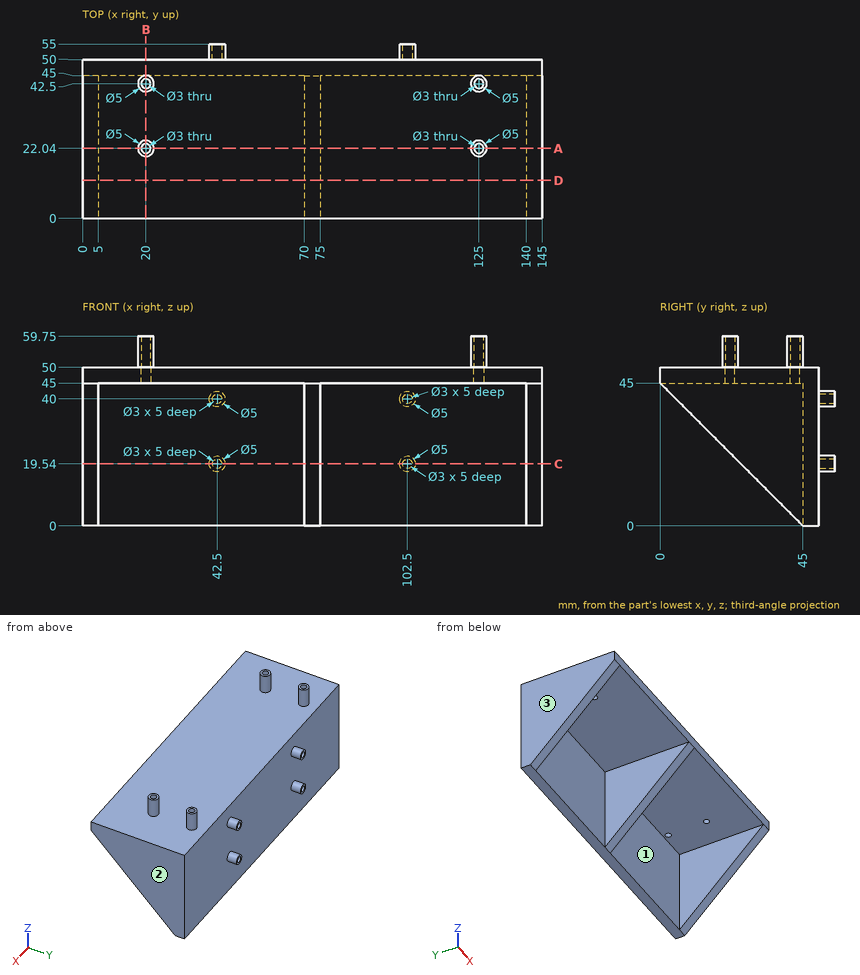
Job drawing, mm, ordinate dimensions from the low corner. One solid piece. Coordinates: 2 decimals unless noted, no trailing zeros. Order: outer loops, then holes, each group sorted by start corner. A loop starts at its lowest first (then second) coordinate and runs counter-clockwise, first axis right, second up. Notation, with made-up numbers: M 51,-35 L 57,-35 A35 cw 57,-3 Z; hole C -9,87 d11. An arc over 180 degrees is marked long. One line per question, with ' | ' between items.
Q1. Slice it at A-A (y = 22.04). Give the cut face in (x, z).
A:
outline: M 0,22.96 L 5,22.96 L 5,45 L 18.5,45 L 18.5,59.75 L 17.5,59.75 L 17.5,50 L 0,50 Z; M 21.5,45 L 70,45 L 70,22.96 L 75,22.96 L 75,45 L 123.5,45 L 123.5,59.75 L 122.5,59.75 L 122.5,50 L 22.5,50 L 22.5,59.75 L 21.5,59.75 Z; M 126.5,45 L 140,45 L 140,22.96 L 145,22.96 L 145,50 L 127.5,50 L 127.5,59.75 L 126.5,59.75 Z
Q2. Slice it at C-C (z = 19.54). Give the cut face in (x, y), and give its area (3 significant figures).
A:
outline: M 0,25.46 L 5,25.46 L 5,45 L 70,45 L 70,25.46 L 75,25.46 L 75,45 L 140,45 L 140,25.46 L 145,25.46 L 145,50 L 105,50 L 105,55 L 104,55 L 104,50 L 101,50 L 101,55 L 100,55 L 100,50 L 45,50 L 45,55 L 44,55 L 44,50 L 41,50 L 41,55 L 40,55 L 40,50 L 0,50 Z | area: 1,040 mm^2
Q3. Drill centre lines: line 1 (Y direction, x = 125, z = 54); line 2 (Y direction, x = 125, z = 48); line 3 (X direction, y = 34, z = 31). Where is each one in solid material? Low to high.
A:
line 1: y = 19.54 to 20.54, 23.54 to 24.54, 40 to 41, 44 to 45 | line 2: y = 0 to 20.54, 23.54 to 41, 44 to 50 | line 3: x = 0 to 5, 70 to 75, 140 to 145
Q4. Slice it at B-B (x = 20). Give the cut face in (y, z), and give its area (3 significant figures).
A:
outline: M 0,45 L 20.54,45 L 20.54,59.75 L 19.54,59.75 L 19.54,50 L 0,50 Z; M 23.54,45 L 41,45 L 41,59.75 L 40,59.75 L 40,50 L 24.54,50 L 24.54,59.75 L 23.54,59.75 Z; M 44,45 L 45,45 L 45,0 L 50,0 L 50,50 L 45,50 L 45,59.75 L 44,59.75 Z | area: 484 mm^2
Q5. Two-plate mould, pull along X, no slides. Class the marked faces 1, 2 and 3: +X half, -X half, draft (parallel to the pull), parting line (faces both ways), or undercut.
A:
face 1: undercut | face 2: +X half | face 3: -X half
Q6. Slice it at D-D (y = 12). Give the cut face in (x, z).
A:
outline: M 0,33 L 5,33 L 5,45 L 70,45 L 70,33 L 75,33 L 75,45 L 140,45 L 140,33 L 145,33 L 145,50 L 0,50 Z
Q7. Pin check, flat tips, straight feed: P1, Ø15, axis at x = 97.5, y = 17.5, coming from the +Z side; P2, Ø5, axis at x = 125, y = 22.04, coming from the -Z side; P3, Ø10, axis at x = 27, z = 17.5, coming from the -Y side; P4, Ø2.5, axis at x = 20, y = 42.5, coming from the -Z side. Stop position of each tip, or through.
A:
P1: stops at z = 50 | P2: stops at z = 45 | P3: stops at y = 45 | P4: passes through
